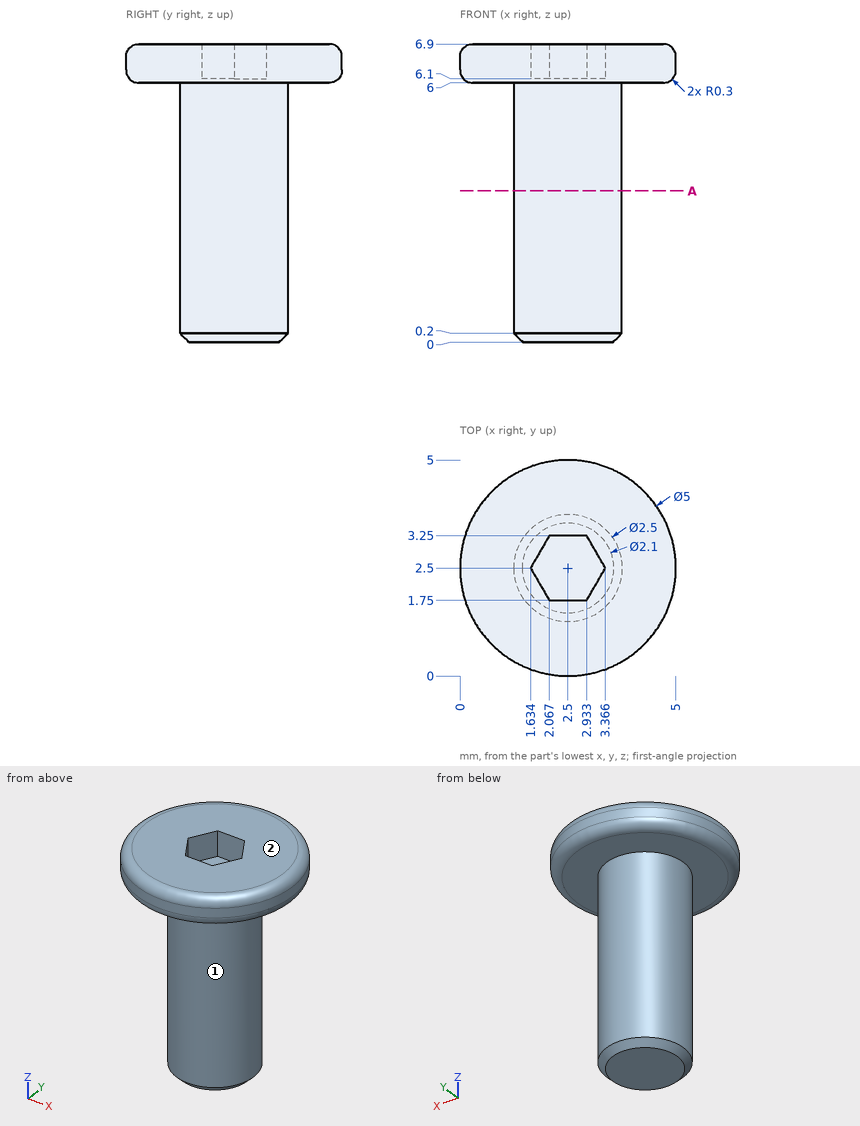
Source: three-view drawing plus pictorial views. Frame: mm from the lowest corner of the part. A direction names the side the tool comes from. Coordinates: 2 decimals unless noted, no trailing zeros. Write each loop counter-clockwise with the first axis right and the second up, starting at its lowest first coordinate (ties: lowest second). Pieces come first, ordered by that corner, then holes. Notation, with made-up numbers: (-2, 79.5) - (23, 79.5) arc R23 ccw to (23, 116.5) - close; hole circle Ø11 at (-19, 88). An arc over 180 degrees is marked (long way). Return JSON: item names as keys, results as strings.
Item 1: Reachability of the marked faces 1 and 2 from +Z, -Z, +X, -X, +Y, -Y: full face, straight path, thin tool, end or side. Return the list, or none.
Completed:
{"face 1": "-Z", "face 2": "+Z, +X, -X, +Y, -Y"}
Item 2: Section query A-A (z = 3.5). Output: boundary loops of the cut face in (x, y).
Completed:
{"outline": "circle Ø2.5 at (2.5, 2.5)"}
Item 3: Pin query (flat end, axial travel): pin 1 Ø1.5 at (x, z) = (1.5, 4) entering from +Y; pin 2 Ø0.8 at (x, y) = (2.5, 2.5) entering from +Z; pin 3 Ø1.5 at (y, z) = (4, 5.5) entering from +X. Return the tip coordinate at first contact, or that it passes through.
Completed:
{"pin 1": "stops at y = 3.72", "pin 2": "stops at z = 6.1", "pin 3": "stops at x = 4.69"}
Item 4: Line query: L1, parallel to X at y = 2.55, z = 4.5; L2, parallel to Z at x = 2.65, y = 2.35; L3, parallel to Z at x = 4.6, y = 2.4. Output: solid intervals per line, ascending.
Completed:
{"L1": "x = 1.25 to 3.75", "L2": "z = 0 to 6.1", "L3": "z = 6 to 6.9"}
